from build123d import *

# Parameters (mm, degrees)
SKETCH2_R           = 10
SKETCH2_R_2         = 1.05
SKETCH2_R_3         = 4.25
BOSS_EXTRUDE2_DEPTH = 3.25


with BuildPart() as part:
    # Sketch2 → Boss-Extrude2 (new body)
    # profile 1 of 2: a face of its own
    with BuildSketch(Plane.XY):
        with BuildLine():
            Line((-24, 0), (-10, 0))
            ThreePointArc((-10, 0), (-9.17454943, 3.978397008), (-6.83447145, 7.3))
            Line((-6.83447145, 7.3), (-16.7, 7.3))
            ThreePointArc((-16.7, 7.3), (-21.861879503, 5.161879503), (-24, 0))
        make_face()
    # profile 2 of 2: a face of its own
    with BuildSketch(Plane.XY):
        Circle(SKETCH2_R)
        with Locations(Location((0, -7, 0), (0, 0, 180))):
            Circle(SKETCH2_R_2, mode=Mode.SUBTRACT)
        with Locations(Location((-7, 0, 0), (0, 0, 180))):
            Circle(SKETCH2_R_2, mode=Mode.SUBTRACT)
        with Locations(Location((0, 7, 0), (0, 0, 180))):
            Circle(SKETCH2_R_2, mode=Mode.SUBTRACT)
        with Locations(Location((7, 0, 0), (0, 0, 180))):
            Circle(SKETCH2_R_2, mode=Mode.SUBTRACT)
        with Locations(Location((0, 0, 0), (0, 0, 180))):
            Circle(SKETCH2_R_3, mode=Mode.SUBTRACT)
    extrude(amount=BOSS_EXTRUDE2_DEPTH)


solid = part.part
Geometry: final body of the model. Coordinates: model frame, mm. A direction names the side the tool comes from. Give positions to 0.01 mm unless a question says otherwise; leave off trailing zeros. Order: outer loops, then holes, each group sorted by start corner. A loop starts at its lowest first (then second) coordinate and runs counter-clockwise, first axis right, second up. Notation, with made-up numbers: (53.25, 19) -> (85.25, 19) arc R29 ccw to (85.25, 52) -> close; hole circle Ø10 at (36, 31). An arc over 180 degrees is marked (long way). Write each question's results on one line, items separated by ' | '.
1) Line query: line 1 along Y through (x, z) = (0, 2.3); line 2 along X through (y, z) = (-2.25, 3.15); line 3 along Y through (x, z) = (7, 2.1). Output: solid intervals per line, ascending.
Geometry says:
line 1: y = -10 to -8.05, -5.95 to -4.25, 4.25 to 5.95, 8.05 to 10 | line 2: x = -9.74 to -3.61, 3.61 to 9.74 | line 3: y = -7.14 to -1.05, 1.05 to 7.14
2) First-contact query: pin 1 Ø1.6 at (x, z) = (-19, 1) entering from -Y; pin 2 Ø1 at (x, z) = (4, 2) entering from -Y; pin 3 Ø1.7 at (x, y) = (0, 7) entering from +Z. Flat tips, straight axial feed; report the tip coordinate or a pass-through.
Geometry says:
pin 1: stops at y = 0 | pin 2: stops at y = -9.37 | pin 3: passes through
3) Set-up query: faces 4 (the face through (-12, 7.3, 2)), 5 (the face through (-0.56, 6.11, 1.6)). Return all of +Z, -Z, +X, -X, +Y, -Y with unobstructed straight access to the full face (end or side cutting, diameter ignored); none if empty.
Geometry says:
face 4: +Z, -Z, -X, +Y | face 5: +Z, -Z
4) Cut plane C-C (y = -7). Output: boundary loops of the cut face in (x, z), and give its area (3 significant figures).
Geometry says:
outline: (-7.14, 0) -> (-1.05, 0) -> (-1.05, 3.25) -> (-7.14, 3.25) -> close; (1.05, 0) -> (7.14, 0) -> (7.14, 3.25) -> (1.05, 3.25) -> close | area: 39.6 mm²
5) Cut plane A-A (x = 0). Output: boundary loops of the cut face in (y, z).
Geometry says:
outline: (-10, 0) -> (-8.05, 0) -> (-8.05, 3.25) -> (-10, 3.25) -> close; (-5.95, 0) -> (-4.25, 0) -> (-4.25, 3.25) -> (-5.95, 3.25) -> close; (4.25, 0) -> (5.95, 0) -> (5.95, 3.25) -> (4.25, 3.25) -> close; (8.05, 0) -> (10, 0) -> (10, 3.25) -> (8.05, 3.25) -> close
6) Cut plane B-B (z = 2.35). Output: boundary loops of the cut face in (x, y), and give its area (3 significant figures).
Geometry says:
outline: (-24, 0) -> (-10, 0) arc R10 ccw (long way) to (-6.83, 7.3) -> (-16.7, 7.3) arc R7.3 ccw to start; hole circle Ø2.1 at (-7, 0); hole circle Ø8.5 at (0, 0); hole circle Ø2.1 at (0, -7); hole circle Ø2.1 at (0, 7); hole circle Ø2.1 at (7, 0) | area: 341 mm²
7) Draft query along X for faces 1 (the face through (8.05, -0.05, 1.6)), 2 (the face through (-17, 0, 2)), 3 (the face through (9.016, -4.326, 1.602)). Return one class per face: released by +X, released by -X, zero draft, split by the parting line, or undercut.
Geometry says:
face 1: undercut | face 2: zero draft | face 3: split by the parting line
